```python
from build123d import *

# Parameters (mm, degrees)
SKETCH1_R          = 1.45
SKETCH1_W          = 9.85
SKETCH1_H          = 9.7
MAINLAYOUT_DEPTH   = 10
TSLOT_DEPTH        = 53.936282454
SKETCH3_R          = 4
CUT_EXTRUDE1_DEPTH = 53.936282454


with BuildPart() as part:
    # Sketch1 → MainLayout (new body)
    with BuildSketch(Plane(origin=(0, 0, 0), x_dir=(1, 0, 0), z_dir=(0, 1, 0))):
        with BuildLine():
            Line((-34.5, 31), (0, 31))
            Line((0, 31), (0, 16.25))
            ThreePointArc((0, 16.25), (-11.25, 5), (0, -6.25))
            Line((0, -6.25), (0, -8.5))
            ThreePointArc((0, -8.5), (-4, -12.5), (0, -16.5))
            Line((0, -16.5), (0, -26))
            Line((0, -26), (-15, -26))
            Line((-15, -26), (-15, -36))
            Line((-15, -36), (-25, -36))
            Line((-25, -36), (-25, -26))
            Line((-25, -26), (-37.5, -26))
            Line((-37.5, -26), (-37.5, 28))
            ThreePointArc((-37.5, 28), (-36.621320344, 30.121320344), (-34.5, 31))
        make_face()
        with Locations(Location((-15.5, 20.5, 0), (0, 0, 90))):
            Circle(SKETCH1_R, mode=Mode.SUBTRACT)
        with Locations(Location((-15.5, -10.5, 0), (0, 0, 270))):
            Circle(SKETCH1_R, mode=Mode.SUBTRACT)
        with Locations(Location((-30, 2.2, 0), (0, 0, 270))):
            Circle(SKETCH1_R, mode=Mode.SUBTRACT)
        with Locations((-30, 13.2)):
            Rectangle(SKETCH1_W, SKETCH1_H, mode=Mode.SUBTRACT)
        with Locations((-30, -8.8)):
            Rectangle(SKETCH1_W, SKETCH1_H, mode=Mode.SUBTRACT)
    mainlayout = extrude(amount=MAINLAYOUT_DEPTH)

    # Sketch2 → TSlot (cut, through all)
    with BuildSketch(Plane(origin=(0, 10, 0), x_dir=(1, 0, 0), z_dir=(0, 1, 0))):
        with BuildLine():
            Line((-28.45, -21.5), (-28.45, -26))
            Line((-28.45, -26), (-31.55, -26))
            Line((-31.55, -26), (-31.55, -21.5))
            Line((-31.55, -21.5), (-32.5, -21.5))
            ThreePointArc((-32.5, -21.5), (-32.853553391, -21.353553391), (-33, -21))
            Line((-33, -21), (-33, -18.5))
            ThreePointArc((-33, -18.5), (-32.853553391, -18.146446609), (-32.5, -18))
            Line((-32.5, -18), (-31.55, -18))
            Line((-31.55, -18), (-31.55, -15))
            Line((-31.55, -15), (-28.45, -15))
            Line((-28.45, -15), (-28.45, -18))
            Line((-28.45, -18), (-27.5, -18))
            ThreePointArc((-27.5, -18), (-27.146446609, -18.146446609), (-27, -18.5))
            Line((-27, -18.5), (-27, -21))
            ThreePointArc((-27, -21), (-27.146446609, -21.353553391), (-27.5, -21.5))
            Line((-27.5, -21.5), (-28.45, -21.5))
        make_face()
    tslot = extrude(amount=-TSLOT_DEPTH, mode=Mode.SUBTRACT)

    # Mirror1: MainLayout, TSlot across plane
    add(mainlayout.mirror(Plane(origin=(0, 0, 0), x_dir=(0, 0, 1), z_dir=(1, 0, 0))))
    add(tslot.mirror(Plane(origin=(0, 0, 0), x_dir=(0, 0, 1), z_dir=(1, 0, 0))), mode=Mode.SUBTRACT)

    # Sketch3 → Cut-Extrude1 (cut, through all)
    with BuildSketch(Plane(origin=(0, 10, 0), x_dir=(1, 0, 0), z_dir=(0, 1, 0))):
        with Locations(Location((0, 22.5, 0), (0, 0, 270))):
            Circle(SKETCH3_R)
    extrude(amount=-CUT_EXTRUDE1_DEPTH, mode=Mode.SUBTRACT)


solid = part.part
```
CAD build for the part. Positions are in the model's coordinates, mm. A direction names the side the tool comes from. Round coordinates to 2 decimals unless told otherwise and drop trailing zeros. Order: outer loops, then holes, each group sorted by start corner. A loop starts at its lowest first (then second) coordinate and runs counter-clockwise, first axis right, second up.
Q1. Drop flat-ended pins along their axis: pin 1 (2 mm diameter, centred on x = -11.5, y = 9, fed in from +Z); pin 2 (1.5 mm diameter, centred on x = -8.5, z = -1.5, fed in from -Y). Give the stop position or say it passes through.
Q2. Slice it at D-D (y = 3.5). State how many separate pieces and enclosed holes the cut face has, and give its area (3 significant figures).
Q3. Two-plate mould, pull along Z, no slides. Class faces 1 (the flat face through (28.45, 5, 16)), 2 (the flat face through (30, 5, 3.95)), 3 (the flat face through (20, 5, 36)): pulls with the +Z half, pulls with the -Z half, needs draft (parallel to the pull), parting line crosses it, or undercut.
Q4. Slice it at C-C (z = 2.5). Write the cut outline in (x, y), and give its area (3 significant figures).
Q5. Slice it at B-B (x = 30). Write the cut outline in (y, z), and give its area (3 significant figures).
Q6. Which spindle directions (+Z, -Z, +X, -X, +Y, -Y) get a long thin tool onto all of the face, cutting with end or side? Do faces 4 (the flat face through (30, 5, -18.05)), 5 (the flat face through (34, 5, 26)), 6 (the flat face through (-9, 10, 2)), 7 (the flat face through (-25, 5, 31)), 8 (the flat face through (31.55, 5, 17)). Say none if no direction does.
Q7. Slice it at A-A (z = 24). Write the cut outline in (x, y).
Q8. Wall check: L1, parallel to X at y = 2, z = 8 (3 decimals); L2, parallel to X at y = 4.5, z = 21; L3, parallel to X at y = 6.75, z = 10.5 (3 decimals). Give the ranges that are in metal, low to high.
Results below:
1. pin 1: stops at z = 26
1. pin 2: passes through
2. separate pieces: 1
2. enclosed holes: 13
2. area: 3,460 mm2
3. face 1: needs draft
3. face 2: undercut
3. face 3: pulls with the +Z half
4. outline: (-37.5, 0) - (-8.39, 0) - (-8.39, 10) - (-37.5, 10) - close; (8.39, 0) - (37.5, 0) - (37.5, 10) - (8.39, 10) - close
4. area: 582 mm2
5. outline: (0, -31) - (10, -31) - (10, -18.05) - (0, -18.05) - close; (0, -8.35) - (10, -8.35) - (10, -3.65) - (0, -3.65) - close; (0, -0.75) - (10, -0.75) - (10, 3.95) - (0, 3.95) - close; (0, 13.65) - (10, 13.65) - (10, 15) - (0, 15) - close
5. area: 237 mm2
6. face 4: +Y, -Y
6. face 5: +Z, +X, +Y, -Y
6. face 6: +Z, -Z, +X, -X, +Y
6. face 7: +Z, -X, +Y, -Y
6. face 8: +Z, +Y, -Y
7. outline: (-37.5, 0) - (-31.55, 0) - (-31.55, 10) - (-37.5, 10) - close; (-28.45, 0) - (28.45, 0) - (28.45, 10) - (-28.45, 10) - close; (31.55, 0) - (37.5, 0) - (37.5, 10) - (31.55, 10) - close
8. L1: x = -37.5 to -34.925, -25.075 to 25.075, 34.925 to 37.5
8. L2: x = -37.5 to -33, -27 to 27, 33 to 37.5
8. L3: x = -37.5 to -34.925, -25.075 to -16.95, -14.05 to -3.464, 3.464 to 14.05, 16.95 to 25.075, 34.925 to 37.5
